Input: part model. Units: mm. Frame: model coordinates. Face numbers are marked on the shaded views. A direction names the side the tool comes from. Round coordinates to 2 decimals unless told otherwise and drop trailing zeros. Loops run counter-clockwise (first coordinate to the right, second up) from the corner with the lowest first, then second, coordinate; pieces in that order, holes last.
(1) Cut plane D-D, the plane z = 3. Give the number of separate pieces and of enclosed holes in the cut face, and give its area (3 significant figures).
(2) Cut plane A-A, the plane x = 0. Output: boundary loops of the cut face in (y, z).
(3) Cut plane B-B, the plane z = -2. Output: boundary loops of the cut face in (x, y), and give its area (3 significant figures).
(4) Cut plane C-C, the plane y = 22.75. Output: boundary loops of the cut face in (x, z).
(5) Access query for the marked faces 4 and 5. Directions: +Z, -Z, +X, -X, +Y, -Y. A direction counts if a zero-diameter tool reaches every point of the face in a straight line with its end or side. Return the directions, or none.
(6) Draft query along X for the marked faces 1, 2 and 3. Return one class per face: released by +X, released by -X, zero draft, split by the parting line, or undercut.
(7) Line query: line 1 (Y direction, x = 17.5, z = 3); line 2 (Y direction, x = -18.85, z = 3); line 3 (X direction, y = 1.5, z = 5.25). Output: solid intervals per line, ascending.
(8) First-contact query: pin 1 Ø1.9 at (y, z) = (0, 3) entering from -X; pin 2 Ø5.5 at (y, z) = (0, 3) entering from +X; pin 3 Ø4 at (y, z) = (-8, 3) entering from +X; pin 4 Ø7.5 at (x, y) = (0, 22.75) entering from +Z. Flat tips, straight axial feed; report the tip coordinate or a pass-through.
from build123d import *

# Parameters (mm, degrees)
ESBO_O1_W                                            = 32.5
ESBO_O1_H                                            = 40.5
RESSALTO_EXTRUS_O1_DEPTH                             = 3
ESBO_O4_W                                            = 9.25
ESBO_O4_H                                            = 22.5
RESSALTO_EXTRUS_O2_DEPTH                             = 3
ESBO_O5_R                                            = 4.25
CORTE_EXTRUS_O1_DEPTH                                = 1.5
ESBO_O6_R                                            = 3.25
CORTE_EXTRUS_O2_DEPTH                                = 37.217226564
REBAIXO_PARA_PARAFUSO_COM_CABE_A_REDONDA_D           = 2.4
REBAIXO_PARA_PARAFUSO_COM_CABE_A_REDONDA_DEPTH       = 3
REBAIXO_PARA_PARAFUSO_COM_CABE_A_REDONDA_CBORE_D     = 4.4
REBAIXO_PARA_PARAFUSO_COM_CABE_A_REDONDA_CBORE_DEPTH = 0.7


with BuildPart() as part:
    # Esboço1 → Ressalto-extrusão1 (new body)
    with BuildSketch(Plane.XY):
        with Locations((0, 9)):
            Rectangle(ESBO_O1_W, ESBO_O1_H)
    extrude(amount=-RESSALTO_EXTRUS_O1_DEPTH)

    # Esboço4 → Ressalto-extrusão2 (add)
    with BuildSketch(Plane.ZY.offset(16.25)):
        with Locations((1.625, 0)):
            Rectangle(ESBO_O4_W, ESBO_O4_H)
    ressalto_extrus_o2 = extrude(amount=RESSALTO_EXTRUS_O2_DEPTH)

    # Espelhar1: Ressalto-extrusão2 across plane
    add(ressalto_extrus_o2.mirror(Plane(origin=(0, 0, 0), x_dir=(0, 0, 1), z_dir=(1, 0, 0))))

    # Esboço5 → Corte-extrusão1 (cut)
    with BuildSketch(Plane(origin=(0, 0, -3), x_dir=(-1, 0, 0), z_dir=(0, 0, -1))):
        with Locations((0, 22.75)):
            Circle(ESBO_O5_R)
    extrude(amount=-CORTE_EXTRUS_O1_DEPTH, mode=Mode.SUBTRACT)

    # Esboço6 → Corte-extrusão2 (cut, through all)
    with BuildSketch(Plane(origin=(0, 0, -3), x_dir=(-1, 0, 0), z_dir=(0, 0, -1))):
        with Locations(Location((0, 22.75, 0), (0, 0, 180))):
            Circle(ESBO_O6_R)
    extrude(amount=-CORTE_EXTRUS_O2_DEPTH, mode=Mode.SUBTRACT)

    # Rebaixo para parafuso com cabeça redonda de M21
    with Locations(Plane.ZY.offset(19.25)):
        with Locations((3, 8), (3, 0), (3, -8)):
            rebaixo_para_parafuso_com_cabe_a_redonda = CounterBoreHole(REBAIXO_PARA_PARAFUSO_COM_CABE_A_REDONDA_D / 2, REBAIXO_PARA_PARAFUSO_COM_CABE_A_REDONDA_CBORE_D / 2, REBAIXO_PARA_PARAFUSO_COM_CABE_A_REDONDA_CBORE_DEPTH, depth=REBAIXO_PARA_PARAFUSO_COM_CABE_A_REDONDA_DEPTH)

    # Espelhar3: Rebaixo para parafuso com cabeça redonda de M21 across plane
    add(rebaixo_para_parafuso_com_cabe_a_redonda.mirror(Plane(origin=(0, 0, 0), x_dir=(0, 0, 1), z_dir=(1, 0, 0))), mode=Mode.SUBTRACT)


solid = part.part
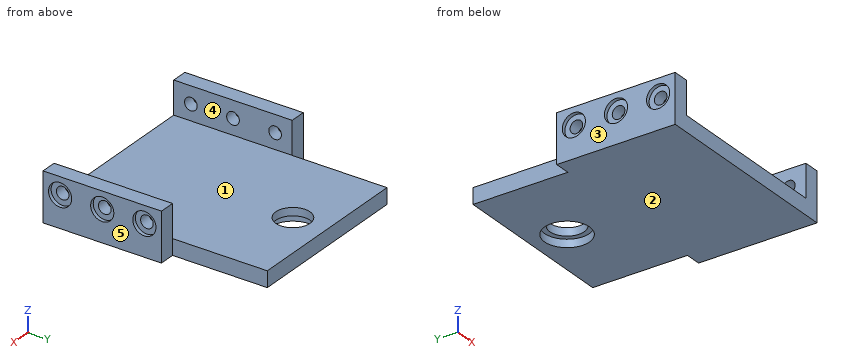
Reported:
1. separate pieces: 8
1. enclosed holes: 0
1. area: 83.4 mm2
2. outline: (-11.25, -3) - (18.5, -3) - (18.5, -1.5) - (19.5, -1.5) - (19.5, 0) - (-11.25, 0) - close; (26, -1.5) - (27, -1.5) - (27, -3) - (29.25, -3) - (29.25, 0) - (26, 0) - close
3. outline: (-19.25, -11.25) - (19.25, -11.25) - (19.25, 11.25) - (16.25, 11.25) - (16.25, 29.25) - (-16.25, 29.25) - (-16.25, 11.25) - (-19.25, 11.25) - close; hole circle Ø8.5 at (0, 22.75)
3. area: 1,390 mm2
4. outline: (-16.25, -3) - (-4.25, -3) - (-4.25, -1.5) - (-3.25, -1.5) - (-3.25, 0) - (-16.25, 0) - close; (3.25, -1.5) - (4.25, -1.5) - (4.25, -3) - (16.25, -3) - (16.25, 0) - (3.25, 0) - close
5. face 4: +Z, +Y, -Y
5. face 5: +Z, -Z, +X, +Y, -Y
6. face 1: undercut
6. face 2: zero draft
6. face 3: released by -X
7. line 1: y = -11.25 to -9.2, -6.8 to -1.2, 1.2 to 6.8, 9.2 to 11.25
7. line 2: y = -11.25 to -10.2, -5.8 to -2.2, 2.2 to 5.8, 10.2 to 11.25
7. line 3: x = -19.25 to -16.25, 16.25 to 19.25
8. pin 1: passes through
8. pin 2: stops at x = 19.25
8. pin 3: stops at x = 18.55
8. pin 4: stops at z = 0
